Study the drawing (mm; zero at the part's minimum x, y, z) and answer. A direction names the side the tool comes from. Round coordinates to 2 decimals unless told otherwise and drop trailing zeros. Write each loop counter-clockwise with the first axis right and the second up, starting at its lowest first coordinate (ties: lowest second). Pieces come first, ordered by that corner, then holes. Notation, with made-up numbers: M 9.5,50.25 L 56.5,50.25 A18 ccw 56.5,72.25 Z; hole C 18.25,40 d2. An arc over 180 degrees is marked long. Put each result on its own line as item: value. Start each with the question number.
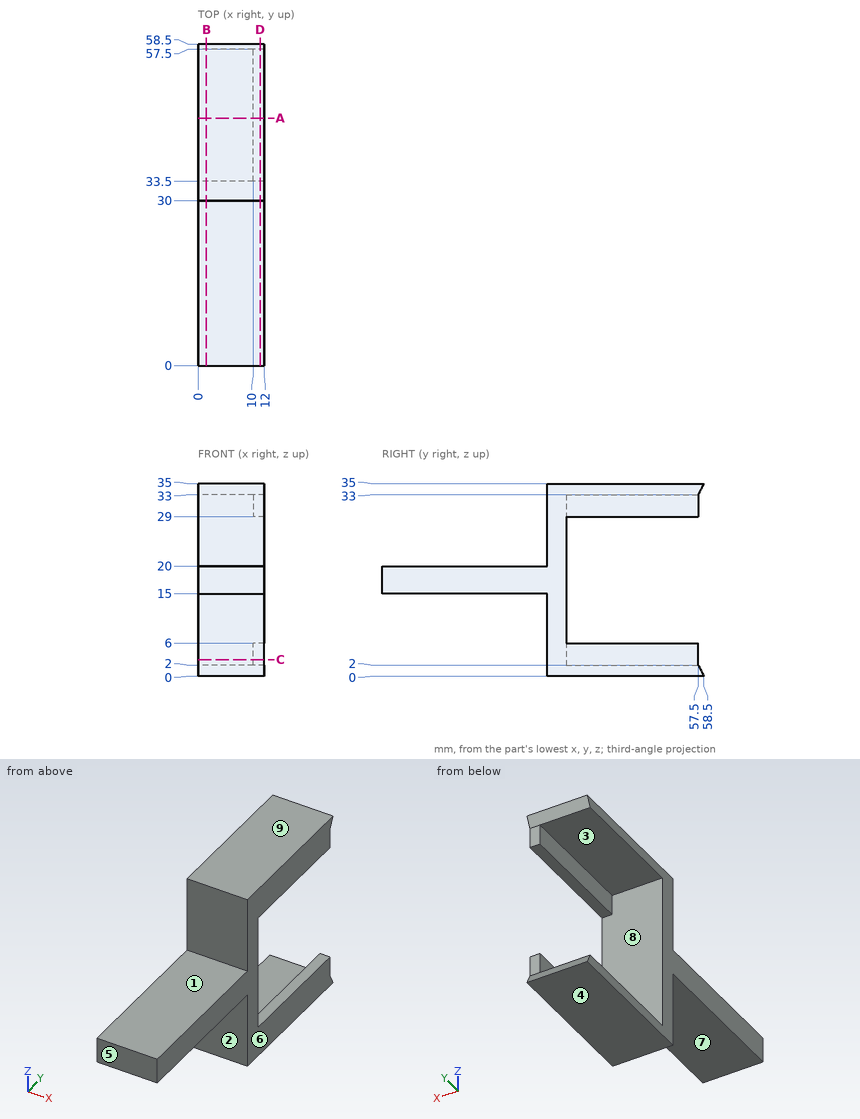
Item 1: Consider line 1 along Z through (x, y) = (10.5, 39); line 2 along Z through (x, y) = (9.5, 44); line 3 along Y through (x, z) = (3, 18). Determine where each line is inside the solid, lowest interval first. Write a range as [from, to].
Item 2: Section C-C (z = 3) is taken. Give the vertices of the cut face in (x, y), and give its area (3 significant figures).
Item 3: Section A-A (y = 45) is taken. Give the vertices of the cut face in (x, z).
Item 4: Determine the mould class of the marked faces 6, 7, 8 and 9 for opening direction Z: released by +Z, released by -Z, zero draft, split by the parting line, or undercut.
Item 5: Flat-ended cylindrical pins translate along their axes: pin 1 (3.5 mm diameter, centred on x = 7.5, y = 15.5, fed in from -Z); pin 2 (3 mm diameter, centred on x = 6.5, z = 29.5, fed in from +Y); pin 3 (0.6 mm diameter, centred on x = 11, z = 30, fed in from +Y). Find the tip coordinate at first contact, or state that the pin passes through.
Item 6: Section D-D (x = 11.25) is taken. Give the vertices of the cut face in (y, z).
Item 7: Which of the six approach directions +Z, -Z, +X, -X, +Y, -Y give full straight-line access (tool end or side, diameter ignored) to the marked faces 1, 2, 3, 4 and 5?
Item 8: Section B-B (x = 1.5) is taken. Give the vertices of the cut face in (y, z), and give its area (4 significant figures).
Output values:
1. line 1: z = [0, 6], [29, 35]
1. line 2: z = [0, 2], [33, 35]
1. line 3: y = [0, 33.5]
2. outline: M 0,30 L 12,30 L 12,57.5 L 10,57.5 L 10,33.5 L 0,33.5 Z
2. area: 90.0 mm^2
3. outline: M 0,0 L 12,0 L 12,6 L 10,6 L 10,2 L 0,2 Z; M 0,33 L 10,33 L 10,29 L 12,29 L 12,35 L 0,35 Z
4. face 6: zero draft
4. face 7: released by -Z
4. face 8: undercut
4. face 9: released by +Z
5. pin 1: stops at z = 15
5. pin 2: stops at y = 33.5
5. pin 3: stops at y = 57.5
6. outline: M 0,15 L 30,15 L 30,0 L 58.5,0 L 57.5,2 L 57.5,6 L 33.5,6 L 33.5,29 L 57.5,29 L 57.5,33 L 58.5,35 L 30,35 L 30,20 L 0,20 Z
7. face 1: +Z, +X, -X, -Y
7. face 2: -Z, +X, -X, -Y
7. face 3: -X, +Y
7. face 4: -Z, +X, -X, +Y, -Y
7. face 5: +Z, -Z, +X, -X, -Y
8. outline: M 0,15 L 30,15 L 30,0 L 58.5,0 L 57.5,2 L 33.5,2 L 33.5,33 L 57.5,33 L 58.5,35 L 30,35 L 30,20 L 0,20 Z
8. area: 370.5 mm^2
